Part model, mm, in its own coordinate system. A direction names the side the tool comes from. Give positions to 0.01 mm unless a question says otherwise; leave off trailing zeros. Write each loop counter-clockwise with the first axis right and the second up, starting at its lowest first coordinate (ties: lowest second). Pieces come first, ordered by that corner, then holes. Notation, with made-up numbers: M -40,-13 L 14,-13 A30 ccw 14,9 Z; hole C 89,-14 d2. An arc over 180 degrees is marked long. Use CSV: the item, a comma, the result in double quotes. Start each with the question number.
Item 1: Pin check, flat tips, straight feed: pin 1 (2 mm diameter, centred on y = 18, z = -5.5, fed in from +X); pin 2 (11 mm diameter, centred on x = 12, z = -5.5, fed in from +Y); pin 3 (0.9 mm diameter, centred on x = 22.5, y = 7.5, fed in from -Z); pin 4 (12 mm diameter, centred on x = 16.5, y = 5, fed in from -Z). Stop position of each tip, or through.
Item 2: Cut at A-A (y = 6.5). List the corners of the cut face in (x, z).
Item 3: Which spindle directions (+Z, -Z, +X, -X, +Y, -Y) get a long thin tool onto all of the face, cutting with end or side? Do faces 1 (the flat face through (17.474, 15.619, -12.976)), 2 (the flat face through (19.9, 21.4, 11.5)), 3 (the cylindrical face through (18.2, 15.6, -10.5)), 4 (the flat face through (8.53, 3.46, -21.75)). Say none if no direction does.
Item 4: Mould opens along Z. For faces 5 (the flat face through (-15.93, 8.84, 17.59)), 6 (the flat face through (14.79, 3.463, -18.596)), 7 (the flat face through (-19.9, 22.16, 11.47)) say: released by +Z, released by -Z, zero draft, split by the parting line, or undercut.
Item 5: Drill centre lines: line 1 (X direction, y = 10.05, z = 0.01); line 2 (Z direction, x = 0, y = 10.25); line 3 (Z direction, x = -4, y = 11.5). Where is each one in solid material? Low to high. Write a range as [from, to].
from build123d import *
from build123d.topology import SkipClean

# Parameters (mm, degrees)
SKETCH_1_R               = 22.5
EXTRUDE_1_DEPTH          = 13.4
SKETCH_2_R               = 2.1
EXTRUDE_2_DEPTH          = 4
FILLET_1_R               = 3.69
EXTRUDE_3_DEPTH          = 9.5
EXTRUDE_START            = -2
EXTRUDE_5_DEPTH          = 2
EXTRUDE_4_DEPTH          = 4.5
CUT_EXTRUDE_START        = -11
SKETCH_5_R               = 21.001588026
CUT_EXTRUDE_1_DEPTH      = 11
SKETCH_6_R               = 8
CUT_EXTRUDE_2_DEPTH      = 3
PATTERN_CIRCULAR_1_COUNT = 3
EXTRUDE_START_2          = -9
EXTRUDE_6_DEPTH          = 9
EXTRUDE_7_DEPTH          = 1
EXTRUDE_8_DEPTH          = 7
CHAMFER_1_SIZE           = 0.5
SKETCH_13_R              = 9.5
CUT_EXTRUDE_4_DEPTH      = 2
EXTRUDE_10_DEPTH         = 13.4
SKETCH_18_W              = 1.5
SKETCH_18_H              = 11.9
EXTRUDE_11_DEPTH         = 0.4


with BuildPart() as part:
    # Эскиз1 → Бобышка-Вытянуть1 (new body)
    with BuildSketch(Plane(origin=(0, 0, 0), x_dir=(1, 0, 0), z_dir=(0, 1, 0))):
        with Locations(Location((0, 0, 0), (0, 0, 270))):
            Circle(SKETCH_1_R)
    extrude(amount=EXTRUDE_1_DEPTH)

    # Эскиз2 → Бобышка-Вытянуть2 (add)
    # profile 1 of 2: a face of its own
    with BuildSketch(Plane.XZ):
        with BuildLine():
            Line((22.193692798, 3.7), (32.5, 3.7))
            Line((32.5, 3.7), (32.5, -3.7))
            Line((32.5, -3.7), (22.193692798, -3.7))
            ThreePointArc((22.193692798, -3.7), (22.5, 0), (22.193692798, 3.7))
        make_face()
        with Locations(Location((28.5, 0, 0), (0, 0, 270))):
            Circle(SKETCH_2_R, mode=Mode.SUBTRACT)
    # profile 2 of 2: a face of its own
    with BuildSketch(Plane.XZ):
        with BuildLine():
            Line((-22.193692798, -3.7), (-32.5, -3.7))
            Line((-32.5, -3.7), (-32.5, 3.7))
            Line((-32.5, 3.7), (-22.193692798, 3.7))
            ThreePointArc((-22.193692798, 3.7), (-22.5, 0), (-22.193692798, -3.7))
        make_face()
        with Locations(Location((-28.5, 0, 0), (0, 0, 90))):
            Circle(SKETCH_2_R, mode=Mode.SUBTRACT)
    extrude(amount=-EXTRUDE_2_DEPTH)

    # Скругление1
    fillet_1_edges = [part.edges().sort_by_distance(p)[0] for p in [
        (-32.5, 2, -3.7),
        (-32.5, 2, 3.7),
        (32.5, 2, 3.7),
        (32.5, 2, -3.7),
    ]]
    fillet(fillet_1_edges, radius=FILLET_1_R)

    # Эскиз3 → Бобышка-Вытянуть3 (add)
    with BuildSketch(Plane(origin=(0, 13.4, 0), x_dir=(1, 0, 0), z_dir=(0, 1, 0))):
        with BuildLine():
            Line((-1, 22.477766793), (-1, 20.977766793))
            ThreePointArc((-1, 20.977766793), (0, 21.001588026), (1, 20.977766793))
            Line((1, 20.977766793), (1, 22.477766793))
            ThreePointArc((1, 22.477766793), (0, 22.5), (-1, 22.477766793))
        make_face()
        with BuildLine():
            Line((19.966317063, -10.372857993), (18.667278957, -9.622857993))
            ThreePointArc((18.667278957, -9.622857993), (18.18790875, -10.500794013), (17.667278957, -11.3549088))
            Line((17.667278957, -11.3549088), (18.966317063, -12.1049088))
            ThreePointArc((18.966317063, -12.1049088), (19.485571585, -11.25), (19.966317063, -10.372857993))
        make_face()
        with BuildLine():
            Line((-18.966317063, -12.1049088), (-17.667278957, -11.3549088))
            ThreePointArc((-17.667278957, -11.3549088), (-18.18790875, -10.500794013), (-18.667278957, -9.622857993))
            Line((-18.667278957, -9.622857993), (-19.966317063, -10.372857993))
            ThreePointArc((-19.966317063, -10.372857993), (-19.485571585, -11.25), (-18.966317063, -12.1049088))
        make_face()
    extrude(amount=EXTRUDE_3_DEPTH)

    # Эскиз7 → Бобышка-Вытянуть5 (add)
    with BuildSketch(Plane.ZY.offset(1).offset(EXTRUDE_START)):
        Polygon((-22.477766793, 22.9), (-23.477766793, 21.4), (-22.477766793, 21.4), align=None)
    extrude_5 = extrude(amount=EXTRUDE_5_DEPTH)

    # Эскиз4 → Бобышка-Вытянуть4 (add)
    with BuildSketch(Plane(origin=(0, 13.4, 0), x_dir=(1, 0, 0), z_dir=(0, 1, 0))):
        with BuildLine():
            Line((-2.5, -20.860679775), (-2.5, -22.360679775))
            ThreePointArc((-2.5, -22.360679775), (0, -22.5), (2.5, -22.360679775))
            Line((2.5, -22.360679775), (2.5, -20.860679775))
            ThreePointArc((2.5, -20.860679775), (0, -21.009949088), (-2.5, -20.860679775))
        make_face()
        with BuildLine():
            Line((-16.815878625, 12.595403397), (-18.114916731, 13.345403397))
            ThreePointArc((-18.114916731, 13.345403397), (-19.485571585, 11.25), (-20.614916731, 9.015276378))
            Line((-20.614916731, 9.015276378), (-19.315878625, 8.265276378))
            ThreePointArc((-19.315878625, 8.265276378), (-18.195149642, 10.504974544), (-16.815878625, 12.595403397))
        make_face()
        with BuildLine():
            Line((19.315878625, 8.265276378), (20.614916731, 9.015276378))
            ThreePointArc((20.614916731, 9.015276378), (19.485571585, 11.25), (18.114916731, 13.345403397))
            Line((18.114916731, 13.345403397), (16.815878625, 12.595403397))
            ThreePointArc((16.815878625, 12.595403397), (18.195149642, 10.504974544), (19.315878625, 8.265276378))
        make_face()
    extrude(amount=EXTRUDE_4_DEPTH)

    # Эскиз5 → Вырез-Вытянуть1 (cut)
    with SkipClean():  # the faces are left unmerged after this step: merging them gives an invalid solid
        with BuildSketch(Plane(origin=(0, 13.4, 0), x_dir=(1, 0, 0), z_dir=(0, 1, 0)).offset(CUT_EXTRUDE_START)):
            with Locations(Location((0, 0, 0), (0, 0, 87.270803902))):
                Circle(SKETCH_5_R)
        extrude(amount=CUT_EXTRUDE_1_DEPTH, mode=Mode.SUBTRACT)

    # Эскиз6 → Вырез-Вытянуть2 (cut)
    with SkipClean():  # the faces are left unmerged after this step: merging them gives an invalid solid
        with BuildSketch(Plane(origin=(0, 0, 0), x_dir=(-1, 0, 0), z_dir=(0, -1, 0))):
            with Locations(Location((0, 0, 0), (0, 0, 90))):
                Circle(SKETCH_6_R)
        extrude(amount=-CUT_EXTRUDE_2_DEPTH, mode=Mode.SUBTRACT)

    # Круговой массив1: Бобышка-Вытянуть5 ×3 about axis
    with SkipClean():  # the faces are left unmerged after this step: merging them gives an invalid solid
        pattern_circular_1_axis = Axis((0, 0, 0), (0, 1, 0))
        for i in range(1, PATTERN_CIRCULAR_1_COUNT):
            add(extrude_5.rotate(pattern_circular_1_axis, i * 360 / PATTERN_CIRCULAR_1_COUNT))

    # Эскиз8 → Бобышка-Вытянуть6 (add)
    with SkipClean():  # the faces are left unmerged after this step: merging them gives an invalid solid
        with BuildSketch(Plane(origin=(0, 13.4, 0), x_dir=(1, 0, 0), z_dir=(0, 1, 0)).offset(EXTRUDE_START_2)):
            with BuildLine():
                Line((7.917321695, 23.713203436), (6.638578465, 21.498355192))
                ThreePointArc((6.638578465, 21.498355192), (11.25, 19.485571585), (15.298832503, 16.498355192))
                Line((15.298832503, 16.498355192), (16.577575733, 18.713203436))
                ThreePointArc((16.577575733, 18.713203436), (12.5, 21.650635095), (7.917321695, 23.713203436))
            make_face()
            with BuildLine():
                Line((-7.917321695, -23.713203436), (-6.638578465, -21.498355192))
                ThreePointArc((-6.638578465, -21.498355192), (-11.25, -19.485571585), (-15.298832503, -16.498355192))
                Line((-15.298832503, -16.498355192), (-16.577575733, -18.713203436))
                ThreePointArc((-16.577575733, -18.713203436), (-12.5, -21.650635095), (-7.917321695, -23.713203436))
            make_face()
        extrude(amount=EXTRUDE_6_DEPTH)

    # Эскиз9 → Бобышка-Вытянуть7 (add)
    with SkipClean():  # the faces are left unmerged after this step: merging them gives an invalid solid
        with BuildSketch(Plane(origin=(0, 13.4, 0), x_dir=(1, 0, 0), z_dir=(0, 1, 0))):
            Polygon((8.069392034, 22.476596989), (7.869392034, 22.130186827), (15.230607966, 17.880186827), (15.430607966, 18.226596989), align=None)
            Polygon((-8.069392034, -22.476596989), (-15.430607966, -18.226596989), (-15.230607966, -17.880186827), (-7.869392034, -22.130186827), align=None)
        extrude(amount=EXTRUDE_7_DEPTH)

    # Эскиз10 → Бобышка-Вытянуть8 (add)
    with SkipClean():  # the faces are left unmerged after this step: merging them gives an invalid solid
        with BuildSketch(Plane(origin=(0, 14.4, 0), x_dir=(1, 0, 0), z_dir=(0, 1, 0))):
            Polygon((10.580865705, 21.026596989), (10.380865705, 20.680186827), (12.719134295, 19.330186827), (12.919134295, 19.676596989), align=None)
            Polygon((-10.580865705, -21.026596989), (-12.919134295, -19.676596989), (-12.719134295, -19.330186827), (-10.380865705, -20.680186827), align=None)
        extrude(amount=EXTRUDE_8_DEPTH)

    # Фаска1
    chamfer_1_edges = [part.edges().sort_by_distance(p)[0] for p in [
        (10.480865705, 21.4, -20.853391908),
        (12.819134295, 21.4, -19.503391908),
        (-10.480865705, 21.4, 20.853391908),
        (-12.819134295, 21.4, 19.503391908),
    ]]
    chamfer(chamfer_1_edges, length=CHAMFER_1_SIZE)

    # Эскиз11 → Повернуть1 (revolve)
    with SkipClean():  # the faces are left unmerged after this step: merging them gives an invalid solid
        with BuildSketch(Plane(origin=(0, 0, 0), x_dir=(0, 0, -1), z_dir=(1, 0, 0))):
            Polygon((20.5, 2.4), (17.5, 2.4), (4.99, 9.622651868), (4.99, 10.9), (15.74, 10.9), (15.74, 11.4), (-0.01, 11.4), (-0.01, 10.9), (4.49, 10.9), (4.49, 9.333976733), (17.366025404, 1.9), (20.5, 1.9), align=None)
        revolve(axis=Axis((0, 0, 0.01), (0, 1, 0)))

    # Эскиз13 → Вырез-Вытянуть4 (cut)
    with SkipClean():  # the faces are left unmerged after this step: merging them gives an invalid solid
        with BuildSketch(Plane.XZ):
            with Locations(Location((0, 0, 0), (0, 0, 270))):
                Circle(SKETCH_13_R)
        extrude(amount=-CUT_EXTRUDE_4_DEPTH, mode=Mode.SUBTRACT)

    # Эскиз15 → Бобышка-Вытянуть10 (add)
    with SkipClean():  # the faces are left unmerged after this step: merging them gives an invalid solid
        with BuildSketch(Plane.XZ):
            with BuildLine():
                Line((-21.937410968, 5), (-22.75, 5))
                Line((-22.75, 5), (-22.75, -5))
                Line((-22.75, -5), (-21.937410968, -5))
                ThreePointArc((-21.937410968, -5), (-22.5, 0), (-21.937410968, 5))
            make_face()
            with BuildLine():
                Line((22.75, 5), (22.75, -5))
                Line((22.75, -5), (21.937410968, -5))
                ThreePointArc((21.937410968, -5), (22.5, 0), (21.937410968, 5))
                Line((21.937410968, 5), (22.75, 5))
            make_face()
        extrude(amount=-EXTRUDE_10_DEPTH)

    # Эскиз18 → Бобышка-Вытянуть11 (add)
    with SkipClean():  # the faces are left unmerged after this step: merging them gives an invalid solid
        with BuildSketch(Plane(origin=(11.75, 0, -20.351596989), x_dir=(-0.8660254037844386, 0, -0.5), z_dir=(0.5000000000000001, 0, -0.8660254037844387))):
            with Locations((-3.5, 8.45)):
                Rectangle(SKETCH_18_W, SKETCH_18_H)
            with Locations((3.5, 8.45)):
                Rectangle(SKETCH_18_W, SKETCH_18_H)
        extrude_11 = extrude(amount=-EXTRUDE_11_DEPTH)

    # Зеркальное отражение1: Бобышка-Вытянуть11 across plane
    with SkipClean():  # the faces are left unmerged after this step: merging them gives an invalid solid
        add(extrude_11.mirror(Plane(origin=(0, 0, 0), x_dir=(0.8660254037844386, 0, 0.5000000000000002), z_dir=(0.5, 0, -0.8660254037844386))))


solid = part.part
Worked answers:
1,pin 1,"passes through"
1,pin 2,"stops at y = 11.4"
1,pin 3,"stops at z = -5"
1,pin 4,"stops at z = -22.69"
2,outline,"M -22.75,-5 L -21.94,-5 A22.5 ccw 6.64,-21.5 L 7.92,-23.71 A25 ccw 16.58,-18.71 L 15.3,-16.5 A22.5 ccw 21.94,-5 L 22.75,-5 L 22.75,5 L 21.94,5 A22.5 ccw -6.64,21.5 L -7.92,23.71 A25 ccw -16.58,18.71 L -15.3,16.5 A22.5 ccw -21.94,5 L -22.75,5 Z; C 0,0.01 d20.82; hole C 0,0 d42; hole C 0,0.01 d18.82"
3,face 1,"-Z, +Y"
3,face 2,"+Z, +X, -Y"
3,face 3,"+Y"
3,face 4,"-Y"
4,face 5,"undercut"
4,face 6,"released by -Z"
4,face 7,"released by +Z"
5,line 1,"x = [-22.75, -21], [-5, -4.5], [4.5, 5], [21, 22.75]"
5,line 2,"z = [-22.5, -21], [-4.99, -4.49], [4.51, 5.01], [21, 22.5]"
5,line 3,"z = [-22.14, -20.62], [20.62, 22.14]"
